Answer from the drawing. Dimensions are ordinates in mm from the lowest x, y and z of the part. A direction names the side the tool comes from. Coordinates: 2 decimals unless noted, no trailing zeros. Order: outer loops, then holes, each group sorted by start corner. A loop starts at its lowest first (then second) coordinate and runs counter-clockwise, first axis right, second up. Notation, with made-up numbers: M 10.25,1.25 L 44.25,1.25 A27 ccw 44.25,27.25 Z; hole C 16,-21.75 d10. An arc over 180 degrees is marked long. Write each question's results on one line, items separated by ' | '.
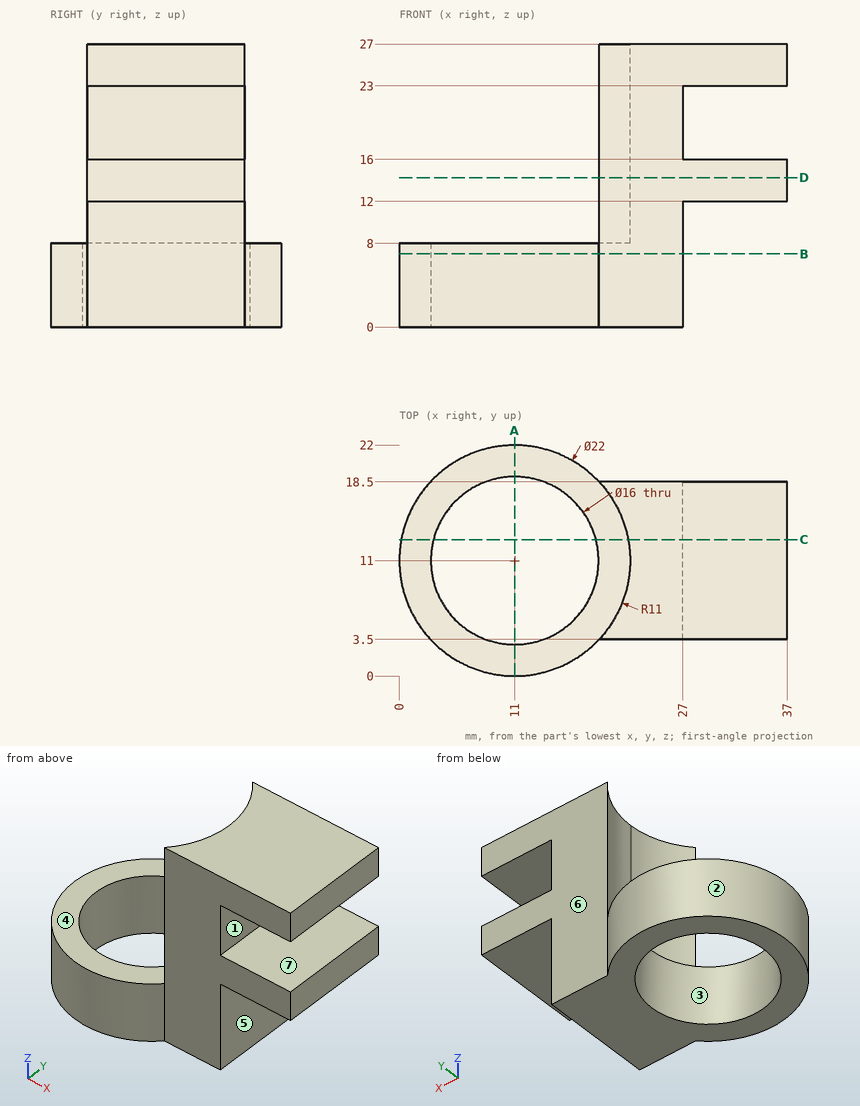
(1) Straight lines are drawn through the part: line 1 (Y direction, x = 11, z = 2); line 2 (Z direction, x = 29, y = 10.5); line 3 (X direction, y = 11, z = 2.75). For each, find the intervals that lie inside material, in ascending order.
Conclusion:
line 1: 0 to 3, 19 to 22 | line 2: 12 to 16, 23 to 27 | line 3: 0 to 3, 19 to 27
(2) For the marked faces 4, 5, 6 and 7, determine the directions among +Z, -Z, +X, -X, +Y, -Y from which every point of the face is accessible in a straight line to the end or side of a thin tool.
Conclusion:
face 4: +Z, -X | face 5: -Z, +X, +Y, -Y | face 6: +Z, -Z, +X, +Y | face 7: +X, +Y, -Y
(3) The part is cut by section B-B, the plane z = 7. Write down the section's boundary in (x, y).
Conclusion:
outline: M 19.05,3.5 L 27,3.5 L 27,18.5 L 19.05,18.5 A11 ccw long Z; hole C 11,11 d16
(4) The part is cut by section D-D, the plane z = 14.25. Write down the section's boundary in (x, y).
Conclusion:
outline: M 19.05,3.5 L 37,3.5 L 37,18.5 L 19.05,18.5 A11 cw 22,11 A11 cw Z
(5) The part is cut by section A-A, the plane x = 11. Write down the section's boundary in (y, z).
Conclusion:
outline: M 0,0 L 3,0 L 3,8 L 0,8 Z; M 19,0 L 22,0 L 22,8 L 19,8 Z
(6) Given pin 1 (2 mm diameter, centred on y = 8, z = 20.5, fed in from +X); pin 2 (10 mm diameter, centred on x = 29, z = 6.5, fed in from -Y); pin 3 (10 mm diameter, centred on x = 7, y = 16, fed in from +Z), each flat-ended and moving along its own axis, determine where each tip first touches the part or whether it passes through.
Conclusion:
pin 1: x = 27 | pin 2: y = 3.5 | pin 3: z = 8
(7) The part is cut by section C-C, the plane y = 13. Write down the section's boundary in (x, z), then the cut area to 3 significant figures.
Conclusion:
outline: M 0.18,0 L 3.25,0 L 3.25,8 L 0.18,8 Z; M 18.75,0 L 27,0 L 27,12 L 37,12 L 37,16 L 27,16 L 27,23 L 37,23 L 37,27 L 21.82,27 L 21.82,8 L 18.75,8 Z | area: 269 mm²
(8) The mould has two halves that part along X. Classify the marked faces 1, 2 and 3: pulls with the +X half, pulls with the -X half, needs draft (parallel to the pull), parting line crosses it, or undercut.
Conclusion:
face 1: pulls with the +X half | face 2: parting line crosses it | face 3: undercut
